Drawing for the job (mm, zero at the part's lowest x, y, z). A direction names the side the tool comes from. Give positions to 0.01 mm unless a question says otherwise; leave off trailing zeros. Loops run counter-clockwise (first coordinate to the right, second up) from the corner with the lowest first, then second, coordinate; pieces in that order, holes last. Notation, with made-up numbers: M 16.25,66 L 75.25,66 A31 cw 75.25,100 Z; hole C 26.25,17.25 d6. An arc over 180 degrees is marked long. Answer in a Markdown table with one row per item. Add a question column.
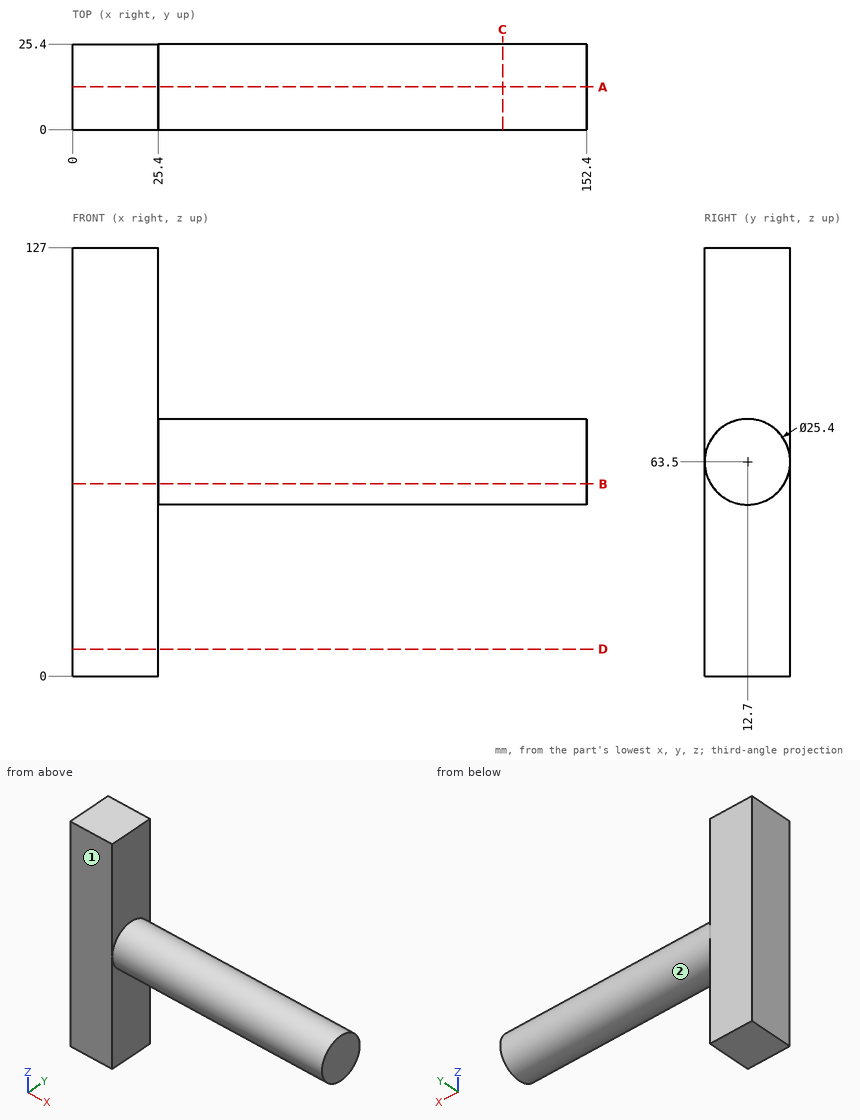
(1) Tool access for the marked faces 1 and 2: list every direction of +Z, -Z, +X, -X, +Y, -Y with a clear straight run to the whole face (end or side of a thin tool).
(2) Wall check: line 1 (X direction, y = 20, z = 106); line 2 (Z direction, x = 98.5, y = 23.5); line 3 (Y direction, x = 42.5, z = 59). Give the ranges that are in metal, low to high.
(3) Slice it at C-C, the plane x = 127.5. Give the cut face in (y, z), then the cut area to 3 significant figures.
(4) Slice it at B-B, the plane z = 57. Give the cut face in (x, y), then the cut area to 3 significant figures.
(5) Slice it at A-A, the plane y = 12.7. Give the cut face in (x, z), then the cut area to 3 significant figures.
(6) Slice it at D-D, the plane z = 8. Give the cut face in (x, y).
(7) Pin check, flat tips, straight feed: pin 1 (8 mm diameter, centred on y = 5.5, z = 15.5, fed in from -X); pin 2 (1 mm diameter, centred on y = 14.5, z = 99, fed in from +X); pin 3 (10 mm diameter, centred on x = 115, y = 21.5, fed in from +Z); pin 4 (1 mm diameter, centred on x = 120, y = 3.5, fed in from +Z). Stop position of each tip, or through.
Solution:
| question | item | result |
|---|---|---|
| 1 | face 1 | +Z, -Z, +X, -X, -Y |
| 1 | face 2 | +X |
| 2 | line 1 | 0 to 25.4 |
| 2 | line 2 | 56.82 to 70.18 |
| 2 | line 3 | 0.82 to 24.58 |
| 3 | outline | C 12.7,63.5 d25.4 |
| 3 | area | 507 mm^2 |
| 4 | outline | M 0,0 L 25.4,0 L 25.4,1.79 L 152.4,1.79 L 152.4,23.61 L 25.4,23.61 L 25.4,25.4 L 0,25.4 Z |
| 4 | area | 3,420 mm^2 |
| 5 | outline | M 0,0 L 25.4,0 L 25.4,50.8 L 152.4,50.8 L 152.4,76.2 L 25.4,76.2 L 25.4,127 L 0,127 Z |
| 5 | area | 6,450 mm^2 |
| 6 | outline | M 0,0 L 25.4,0 L 25.4,25.4 L 0,25.4 Z |
| 7 | pin 1 | x = 0 |
| 7 | pin 2 | x = 25.4 |
| 7 | pin 3 | z = 75.62 |
| 7 | pin 4 | z = 72.75 |
